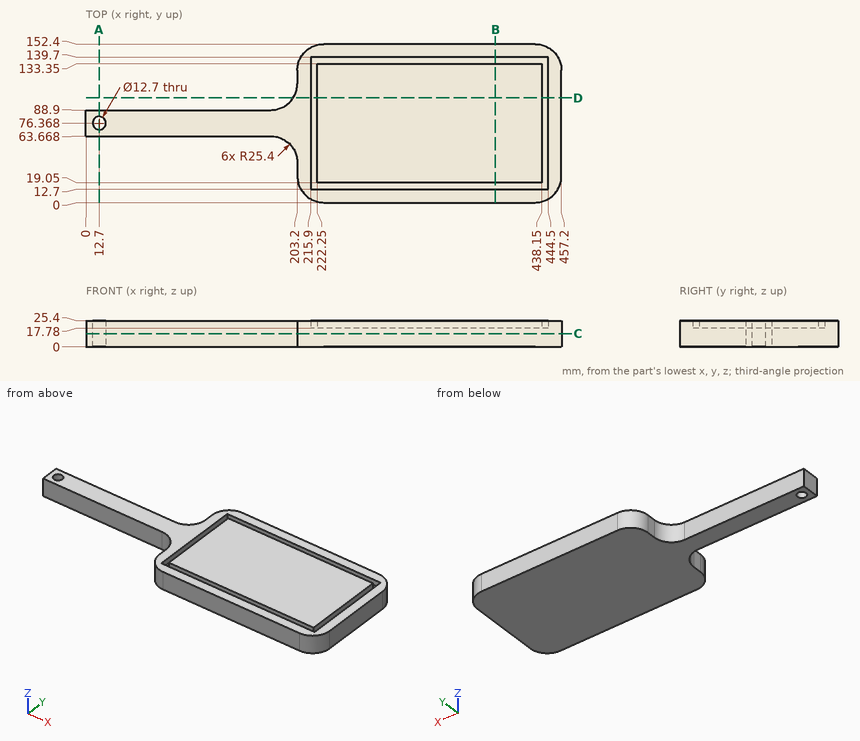
Check sheet for the drawn part. Datum: minimum x, y, z corner. Units: mm. Give positions to 0.01 mm unless a question says otherwise; leave off trailing zeros. Write each loop counter-clockwise with the first axis right and the second up, starting at its lowest first coordinate (ties: lowest second). Pieces come first, ordered by that corner, then holes. Notation, with made-up numbers: (17.25, 74) - (69.25, 74) arc R10 ccw to (69.25, 86) - close; hole circle Ø6 at (1.5, -22). An arc over 180 degrees is marked (long way). Put each result on its own line as item: value.
1. Sectioned sample at A-A, the plane x = 12.7. Enter the section's corners in (y, z).
Ans:
outline: (63.67, 0) - (70.02, 0) - (70.02, 25.4) - (63.67, 25.4) - close; (82.72, 0) - (88.9, 0) - (88.9, 25.4) - (82.72, 25.4) - close
2. Go/stop test with flat-tipped pins: pin 1 (6 mm diameter, centred on x = 269, y = 33.5, fed in from -Z); pin 2 (6 mm diameter, centred on y = 57, z = 19.5, fed in from -X); pin 3 (1 mm diameter, centred on y = 136.5, z = 10.5, fed in from -X); pin 4 (5 mm diameter, centred on x = 180, z = 16.5, fed in from -Y). Record where each tip stops, or that it passes through.
Ans:
pin 1: stops at z = 0
pin 2: stops at x = 190.95
pin 3: stops at x = 204.85
pin 4: stops at y = 63.23
3. Thickness scan on line 1 (Y direction, x = 285, z = 23.5); line 2 (X direction, y = 67.5, z = 22.5); line 3 (Y direction, x = 12.7, z = 18.75). Record the ranges inside material, lowest first.
Ans:
line 1: y = 0 to 12.7, 19.05 to 133.35, 139.7 to 152.4
line 2: x = 0 to 215.9, 222.25 to 438.15, 444.5 to 457.2
line 3: y = 63.67 to 70.02, 82.72 to 88.9
4. Sectioned sample at B-B, the plane x = 393.5. Enter the section's corners in (y, z), plus the area to 3 significant figures.
Ans:
outline: (0, 0) - (152.4, 0) - (152.4, 25.4) - (139.7, 25.4) - (139.7, 17.78) - (133.35, 17.78) - (133.35, 25.4) - (19.05, 25.4) - (19.05, 17.78) - (12.7, 17.78) - (12.7, 25.4) - (0, 25.4) - close
area: 3,770 mm²
5. Sectioned sample at D-D, the plane y = 100.5. Enter the section's corners in (x, z), plus the area to 3 significant figures.
Ans:
outline: (199.12, 0) - (457.2, 0) - (457.2, 25.4) - (444.5, 25.4) - (444.5, 17.78) - (438.15, 17.78) - (438.15, 25.4) - (222.25, 25.4) - (222.25, 17.78) - (215.9, 17.78) - (215.9, 25.4) - (199.12, 25.4) - close
area: 6,460 mm²
6. Sectioned sample at C-C, the plane z = 12.75. Enter the section's corners in (x, y), plus the area to 3 significant figures.
Ans:
outline: (0, 63.67) - (177.8, 63.67) arc R25.4 cw to (203.2, 38.27) - (203.2, 25.4) arc R25.4 ccw to (228.6, 0) - (431.8, 0) arc R25.4 ccw to (457.2, 25.4) - (457.2, 127) arc R25.4 ccw to (431.8, 152.4) - (228.6, 152.4) arc R25.4 ccw to (203.2, 127) - (203.2, 114.3) arc R25.4 cw to (177.8, 88.9) - (0, 88.9) - close; hole circle Ø12.7 at (12.7, 76.37)
area: 43,400 mm²
